The listing builds one solid part. Answer for the finished solid, in the listing's coordinates (mm). A direction names the side the tool comes from. Coordinates: 2 decimals unless noted, no trailing zeros. Write each loop counter-clockwise with the first axis right and the second up, starting at its lowest first coordinate (ties: lowest second). Pieces come first, ordered by that corner, then holes. Notation, with made-up numbers: M -22.75,-18.75 L -18.75,-18.75 A34 cw -18.75,16.25 Z; hole C -20,-34 d8. An arc over 180 degrees is marked long. Answer as CSV lines item,"result". Start each with the question number.
```python
from build123d import *

# Parameters (mm, degrees)
SKETCH_1_R               = 20
EXTRUDE_1_DEPTH          = 3
SKETCH_2_R               = 0.7
CUT_EXTRUDE_1_DEPTH      = 3
PATTERN_CIRCULAR_2_COUNT = 4
SKETCH_4_R               = 2.5
CUT_EXTRUDE_3_DEPTH      = 3
CUT_EXTRUDE_4_DEPTH      = 3
PATTERN_CIRCULAR_4_COUNT = 4


with BuildPart() as part:
    # ｽｹｯﾁ1 → ﾎﾞｽ - 押し出し1 (new body)
    with BuildSketch(Plane.XY):
        Circle(SKETCH_1_R)
    extrude(amount=EXTRUDE_1_DEPTH)

    # ｽｹｯﾁ2 → ｶｯﾄ - 押し出し1 (cut)
    with BuildSketch(Plane.XY.offset(3)):
        with Locations((0, 16)):
            Circle(SKETCH_2_R)
    cut_extrude_1 = extrude(amount=-CUT_EXTRUDE_1_DEPTH, mode=Mode.SUBTRACT)

    # 円形ﾊﾟﾀｰﾝ2: ｶｯﾄ - 押し出し1 ×4 about axis
    pattern_circular_2_axis = Axis((0, 0, 0), (0, 0, 1))
    for i in range(1, PATTERN_CIRCULAR_2_COUNT):
        add(cut_extrude_1.rotate(pattern_circular_2_axis, i * 360 / PATTERN_CIRCULAR_2_COUNT), mode=Mode.SUBTRACT)

    # ｽｹｯﾁ4 → ｶｯﾄ - 押し出し3 (cut)
    with BuildSketch(Plane.XY.offset(3)):
        Circle(SKETCH_4_R)
    extrude(amount=-CUT_EXTRUDE_3_DEPTH, mode=Mode.SUBTRACT)

    # ｽｹｯﾁ5 → ｶｯﾄ - 押し出し4 (cut)
    with BuildSketch(Plane.XY.offset(3)):
        Polygon((4.596194078, 4.596194078), (3.889087297, 5.303300859), (10.960155108, 12.374368671), (12.374368671, 10.960155108), (5.303300859, 3.889087297), align=None)
    cut_extrude_4 = extrude(amount=-CUT_EXTRUDE_4_DEPTH, mode=Mode.SUBTRACT)

    # 円形ﾊﾟﾀｰﾝ4: ｶｯﾄ - 押し出し4 ×4 about axis
    pattern_circular_4_axis = Axis((0, 0, 0), (0, 0, 1))
    for i in range(1, PATTERN_CIRCULAR_4_COUNT):
        add(cut_extrude_4.rotate(pattern_circular_4_axis, i * 360 / PATTERN_CIRCULAR_4_COUNT), mode=Mode.SUBTRACT)


solid = part.part
```
1) Which of the six approach directions +Z, -Z, +X, -X, +Y, -Y give full straight-line access (tool end or side, diameter ignored) to faces 1 (the face through (0, -4, 3)), 2 (the face through (-11.677, 11.657, 1.521))?
2) The part is cut by section D-D (y = 0). Determine the outline of the cut face in (x, z).
3) Find the intervals of material crossed by line 1 (Y direction, x = 0, z = 2.25); line 2 (X direction, y = -6, z = 0.7); line 3 (X direction, y = -5.5, z = 0.8), in increasing order. Write a range as from..to.
4) The part is cut by section C-C (z = 0.85). Count the separate pieces of the cut face and the enclosed holes in it, then the cut area to 3 significant figures.
5) This flat-tipped pin is pushed along its axis until it touches: P1, Ø1, axis at y = -1.5, z = 2.5, coming from the -X side (3 decimals). Where does it stop, or does it pass through?
6) The part is cut by section A-A (y = -16). Determine the outline of the cut face in (x, z).
Completed:
1,face 1,"+Z, +X, -X, +Y, -Y"
1,face 2,"+Z, -Z"
2,outline,"M -20,0 L -16.7,0 L -16.7,3 L -20,3 Z; M -15.3,0 L -2.5,0 L -2.5,3 L -15.3,3 Z; M 2.5,0 L 15.3,0 L 15.3,3 L 2.5,3 Z; M 16.7,0 L 20,0 L 20,3 L 16.7,3 Z"
3,line 1,"-20..-16.7, -15.3..-2.5, 2.5..15.3, 16.7..20"
3,line 2,"-19.08..-7.41, -4.59..4.59, 7.41..19.08"
3,line 3,"-19.23..-6.91, -4.09..4.09, 6.91..19.23"
4,separate pieces,"1"
4,enclosed holes,"9"
4,area,"1,150 mm²"
5,P1,"x = -19.975"
6,outline,"M -12,0 L -0.7,0 L -0.7,3 L -12,3 Z; M 0.7,0 L 12,0 L 12,3 L 0.7,3 Z"
